Can you work these out from the drawing? Everything is in mm from the part's minimum corner. A direction names the side the tool comes from. Round coordinates to 2 decimals unless told otherwise and drop trailing zeros. Loops run counter-clockwise (first coordinate to the right, second up) from the corner with the lowest first, then second, coordinate; pieces in that order, holes last. Notation, with made-up numbers: M -37,46.25 L -2,46.25 A7 ccw -2,56.25 Z; hole C 72,3.5 d11. An arc over 180 degrees is marked long. Use a Markdown table: item, result.
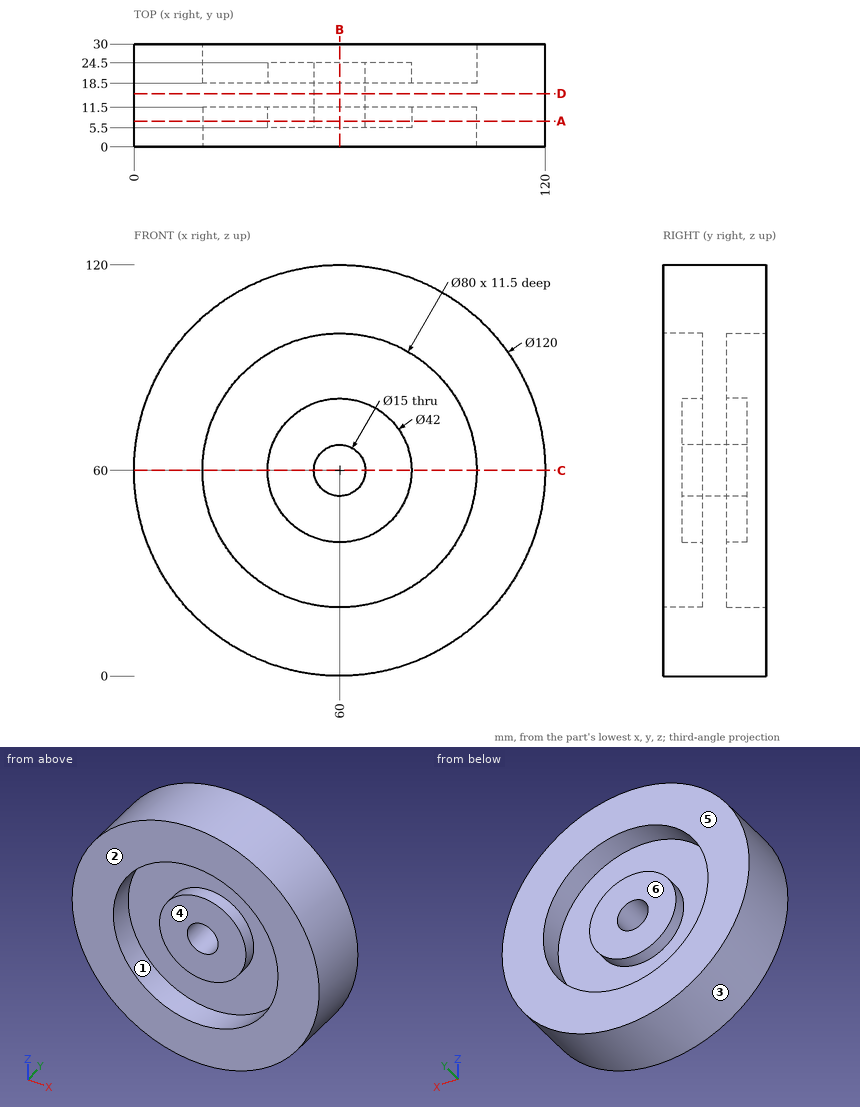
Q1. Imagine slicing it at D-D, the plane y = 15.5. Please give me the cut outline in (x, z), then the cut area to 3 significant figures.
Return value:
| item | result |
|---|---|
| outline | C 60,60 d120; hole C 60,60 d15 |
| area | 11,100 mm^2 |
Q2. Will these pins go through, and if not, where does the flat tip stop? P1, Ø3, axis at x = 82, z = 58, coming from the +Y side; P2, Ø10, axis at y = 11, z = 61.5, coming from the +X side; P3, Ø6, axis at y = 5.5, z = 89, coming from the -X side; P4, Ø24, axis at x = 53, z = 68.5, coming from the -Y side.
Return value:
| item | result |
|---|---|
| P1 | stops at y = 24.5 |
| P2 | stops at x = 120 |
| P3 | stops at x = 5.93 |
| P4 | stops at y = 5.5 |
Q3. Imagine slicing it at B-B, the plane x = 60. Please give me the cut outline in (y, z).
Return value:
| item | result |
|---|---|
| outline | M 0,0 L 30,0 L 30,20 L 18.5,20 L 18.5,39 L 24.5,39 L 24.5,52.5 L 5.5,52.5 L 5.5,39 L 11.5,39 L 11.5,20 L 0,20 Z; M 0,100 L 11.5,100 L 11.5,81 L 5.5,81 L 5.5,67.5 L 24.5,67.5 L 24.5,81 L 18.5,81 L 18.5,100 L 30,100 L 30,120 L 0,120 Z |
Q4. We'd pull the mould along X, two halves only. Please class the marked faces 1, 2 and 3: pulls with the +X half, pulls with the -X half, needs draft (parallel to the pull), parting line crosses it, or undercut.
Return value:
| item | result |
|---|---|
| face 1 | undercut |
| face 2 | needs draft |
| face 3 | parting line crosses it |
Q5. Imagine slicing it at C-C, the plane z = 60. Please give me the cut outline in (x, y), then the cut area to 3 significant figures.
Return value:
| item | result |
|---|---|
| outline | M 0,0 L 20,0 L 20,11.5 L 39,11.5 L 39,5.5 L 52.5,5.5 L 52.5,24.5 L 39,24.5 L 39,18.5 L 20,18.5 L 20,30 L 0,30 Z; M 67.5,5.5 L 81,5.5 L 81,11.5 L 100,11.5 L 100,0 L 120,0 L 120,30 L 100,30 L 100,18.5 L 81,18.5 L 81,24.5 L 67.5,24.5 Z |
| area | 1,980 mm^2 |
Q6. For the marked faces 4, 5 and 6, which set-ups out of +Z, -Z, +X, -X, +Y, -Y let a thin tool reach every point of the face, with its end or its side?
Return value:
| item | result |
|---|---|
| face 4 | -Y |
| face 5 | +Z, -Z, +X, -X, +Y |
| face 6 | +Y |
Q7. I need wall thicknesses on line 1 (Z direction, x = 60, y = 21); line 2 (X direction, y = 19.5, z = 61.5). Which ranges of each line are inside material? Lowest first, please. Write a range as from..to.
Return value:
| item | result |
|---|---|
| line 1 | z = 0..20, 39..52.5, 67.5..81, 100..120 |
| line 2 | x = 0.02..20.03, 39.05..52.65, 67.35..80.95, 99.97..119.98 |
Q8. Imagine slicing it at A-A, the plane y = 7.5. Please give me the cut outline in (x, z).
Return value:
| item | result |
|---|---|
| outline | C 60,60 d120; C 60,60 d42; hole C 60,60 d80; hole C 60,60 d15 |
